```python
from build123d import *

# Parameters (mm, degrees)
SKETCH1_W           = 25.146
SKETCH1_H           = 40.132
SKETCH1_R           = 1.143
BOSS_EXTRUDE1_DEPTH = 1.524
SKETCH2_R           = 10
BOSS_EXTRUDE2_DEPTH = 16.764
SKETCH3_W           = 2.413
SKETCH3_H           = 2.413
BOSS_EXTRUDE3_DEPTH = 1.27
SKETCH4_W           = 0.635
SKETCH4_H           = 0.635
BOSS_EXTRUDE4_DEPTH = 5.842
SKETCH5_W           = 3.348930747
SKETCH5_H           = 5.720091757
BOSS_EXTRUDE5_DEPTH = 3.302


with BuildPart() as part:
    # Sketch1 → Boss-Extrude1 (new body)
    with BuildSketch(Plane(origin=(0, 0, 0), x_dir=(1, 0, 0), z_dir=(0, 1, 0))):
        with Locations((12.573, 20.066)):
            Rectangle(SKETCH1_W, SKETCH1_H)
        with Locations((2.073, 38.066)):
            Circle(SKETCH1_R, mode=Mode.SUBTRACT)
        with Locations((23.073, 38.066)):
            Circle(SKETCH1_R, mode=Mode.SUBTRACT)
        with Locations((23.073, 2.066)):
            Circle(SKETCH1_R, mode=Mode.SUBTRACT)
        with Locations((2.073, 2.066)):
            Circle(SKETCH1_R, mode=Mode.SUBTRACT)
    extrude(amount=BOSS_EXTRUDE1_DEPTH)

    # Sketch2 → Boss-Extrude2 (add)
    with BuildSketch(Plane(origin=(0, 1.524, 0), x_dir=(1, 0, 0), z_dir=(0, 1, 0))):
        with Locations((12.573, 30)):
            Circle(SKETCH2_R)
    extrude(amount=BOSS_EXTRUDE2_DEPTH)

    # Sketch3 → Boss-Extrude3 (add)
    with BuildSketch(Plane(origin=(0, 1.524, 0), x_dir=(1, 0, 0), z_dir=(0, 1, 0))):
        with Locations((7.493, 3.2725)):
            Rectangle(SKETCH3_W, SKETCH3_H)
        with Locations((10.033, 3.2725)):
            Rectangle(SKETCH3_W, SKETCH3_H)
        with Locations((12.573, 3.2725)):
            Rectangle(SKETCH3_W, SKETCH3_H)
        with Locations((15.113, 3.2725)):
            Rectangle(SKETCH3_W, SKETCH3_H)
        with Locations((17.653, 3.2725)):
            Rectangle(SKETCH3_W, SKETCH3_H)
        with Locations((7.493, 5.8125)):
            Rectangle(SKETCH3_W, SKETCH3_H)
        with Locations((10.033, 5.8125)):
            Rectangle(SKETCH3_W, SKETCH3_H)
        with Locations((12.573, 5.8125)):
            Rectangle(SKETCH3_W, SKETCH3_H)
        with Locations((15.113, 5.8125)):
            Rectangle(SKETCH3_W, SKETCH3_H)
        with Locations((17.653, 5.8125)):
            Rectangle(SKETCH3_W, SKETCH3_H)
    extrude(amount=BOSS_EXTRUDE3_DEPTH)

    # Sketch4 → Boss-Extrude4 (add)
    with BuildSketch(Plane(origin=(0, 2.794, 0), x_dir=(1, 0, 0), z_dir=(0, 1, 0))):
        with Locations((10.033, 3.2725)):
            Rectangle(SKETCH4_W, SKETCH4_H)
        with Locations((7.493, 3.2725)):
            Rectangle(SKETCH4_W, SKETCH4_H)
        with Locations((12.573, 3.2725)):
            Rectangle(SKETCH4_W, SKETCH4_H)
        with Locations((15.113, 3.2725)):
            Rectangle(SKETCH4_W, SKETCH4_H)
        with Locations((17.653, 3.2725)):
            Rectangle(SKETCH4_W, SKETCH4_H)
        with Locations((10.033, 5.8125)):
            Rectangle(SKETCH4_W, SKETCH4_H)
        with Locations((12.573, 5.8125)):
            Rectangle(SKETCH4_W, SKETCH4_H)
        with Locations((15.113, 5.8125)):
            Rectangle(SKETCH4_W, SKETCH4_H)
        with Locations((17.653, 5.8125)):
            Rectangle(SKETCH4_W, SKETCH4_H)
        with Locations((7.493, 5.8125)):
            Rectangle(SKETCH4_W, SKETCH4_H)
    extrude(amount=BOSS_EXTRUDE4_DEPTH)

    # Sketch5 → Boss-Extrude5 (add)
    with BuildSketch(Plane.XZ):
        with Locations((3.215733766, -29.18090344)):
            Rectangle(SKETCH5_W, SKETCH5_H)
    extrude(amount=BOSS_EXTRUDE5_DEPTH)


solid = part.part
```
For this review, take the finished solid that the model builds, in its own axes (mm). A direction names the side the tool comes from. Coordinates: 2 decimals unless noted, no trailing zeros. Loops run counter-clockwise (first coordinate to the right, second up) from the corner with the lowest first, then second, coordinate; pieces in that order, holes last. Notation, with made-up numbers: (71, 55) -> (85, 55) arc R31 cw to (85, 85) -> close; hole circle Ø7 at (-16.75, 86.25). An arc over 180 degrees is marked (long way). Return JSON: item names as keys, results as strings. Group by question number.
(1) To check wall thickness, follow L1, parallel to Z at x = 9.75, y = 4.25 (3 decimals); L2, parallel to Z at x = 2.5, y = 0.25; L3, parallel to Y at x = 8, z = -23.5. State the ranges of each line that lie inside material, in increasing order.
(2) Consider section D-D, the plane y = 15.5. Give the boundary of the cut face in (x, z), plus the area to 3 significant figures.
(3) Consider section C-C, the plane y = 5.5. Count the separate pieces of the cut face and the enclosed holes in it, plus the area to 3 significant figures.
(4) Tool access review of faces 1 (the flat face through (6.286, 2, -6)), 2 (the flat face through (7, 2, -2.066)), 3 (the cylindrical face through (2.6, 0.75, -37.05)), 4 (the flat face through (18, 2, -7.019)): name each direction out of +Z, -Z, +X, -X, +Y, -Y from which nothing blocks a thin tool from reaching the whole face with its end or side.
(5) For pin 1 Ø0.6 at (y, z) = (2.5, -3) entering from +X; pin 2 Ø0.5 at (x, y) = (17.5, 5.5) entering from -Z; pin 3 Ø0.7 at (x, z) = (12.5, -5.5) entering from +Y, all flat-tipped, find the tip position at first contact; note any pin that passes through.
(6) Mouldability with a two-part tool opening along X and no side actions: class faces 5 (the cylindrical face through (17.19, 9.79, -21.13)), 6 (the cylindrical face through (22.166, 0.751, -37.371)), 7 (the flat face through (25.146, 1, -20)) as pulls with the +X half, pulls with the -X half, needs draft (parallel to the pull), parting line crosses it, or undercut.
(7) Consider section A-A, the plane z = -30. Give the boundary of the cut face in (x, y).
(8) Consider section B-B, the plane x = 6.75. Give the boundary of the cut face in (y, z), plus the area to 3 significant figures.
Results below:
{
 "1": {"L1": "z = -39.593 to -20.407, -6.13 to -5.495, -3.59 to -2.955", "L2": "z = -40.13 to -39.13, -37.01 to -3.13, -1.01 to 0", "L3": "y = 0 to 18.29"},
 "2": {"outline": "circle Ø20 at (12.57, -30)", "area": "314 mm2"},
 "3": {"separate pieces": "11", "enclosed holes": "0", "area": "318 mm2"},
 "4": {"face 1": "+Z, -X, +Y", "face 2": "+Z, +X, -X, +Y", "face 3": "+Y, -Y", "face 4": "+X, -X, +Y"},
 "5": {"pin 1": "stops at x = 18.86", "pin 2": "stops at z = -38.84", "pin 3": "stops at y = 8.64"},
 "6": {"face 5": "parting line crosses it", "face 6": "undercut", "face 7": "pulls with the +X half"},
 "7": {"outline": "(0, 0) -> (1.54, 0) -> (1.54, -3.3) -> (4.89, -3.3) -> (4.89, 0) -> (25.15, 0) -> (25.15, 1.52) -> (22.57, 1.52) -> (22.57, 18.29) -> (2.57, 18.29) -> (2.57, 1.52) -> (0, 1.52) -> close"},
 "8": {"outline": "(0, -40.13) -> (1.52, -40.13) -> (1.52, -38.13) -> (18.29, -38.13) -> (18.29, -21.87) -> (1.52, -21.87) -> (1.52, -7.02) -> (2.79, -7.02) -> (2.79, -4.61) -> (1.52, -4.61) -> (1.52, -4.48) -> (2.79, -4.48) -> (2.79, -2.07) -> (1.52, -2.07) -> (1.52, 0) -> (0, 0) -> close", "area": "340 mm2"}
}
